Autodesk Inventor part; units mm, degrees
ref_plane "YZ Plane" through (0, 0, 0) normal (1, 0, 0) x (0, 1, 0)
ref_plane "XZ Plane" through (0, 0, 0) normal (0, 1, 0) x (-1, 0, 0)
ref_plane "XY Plane" through (0, 0, 0) normal (0, 0, 1) x (1, 0, 0)
sketch "Эскиз1" plane through (0, 0, 0) normal (0, 0, 1) x (1, 0, 0)
  line L0 (123.2502, 86.3215) -> (123.2502, 112.3215)
  circle A0 centre (130.7502, 114.3215) radius 1.5
  circle A1 centre (130.7502, 84.3215) radius 1.5
  line L1 (132.7502, 121.8215) -> (144.7502, 121.8215)
  arc A2 (132.7502, 121.8215) -> (123.2502, 112.3215) centre (132.7502, 112.3215) ccw
  arc A3 (123.2502, 86.3215) -> (132.7502, 76.8215) centre (132.7502, 86.3215) ccw
  line L2 (138.7502, 76.8215) -> (132.7502, 76.8215)
  line L3 (138.7502, 88.4715) -> (138.7502, 76.8215)
  line L4 (138.7502, 111.4715) -> (138.7502, 98.6715)
  line L5 (144.5002, -126.5097) -> (144.5002, 144.1144)
  line L6 (138.7502, 76.8215) -> (138.7502, 121.8215)
  point P0 (0, 0)
extrude "Выдавливание1" add sketch "Эскиз1" along normal blind 4
fillet "Сопряжение1" radius 2 6 edges at (123.2502, 99.3215, 4) (126.0327, 79.604, 4) (135.7502, 76.8215, 4) (135.7502, 121.8215, 4) (126.0327, 119.039, 4) (138.7502, 99.3215, 4)
fillet "Сопряжение2" radius 2 4 edges at (138.7502, 121.8215, 1) (138.1644, 121.2357, 3.4142) (138.7502, 76.8215, 1) (138.1644, 77.4073, 3.4142)
sketch "Эскиз2" plane through (0, 0, 4) normal (0, 0, 1) x (1, 0, 0)
  circle A0 centre (130.7502, 114.3215) radius 1.5
  line L0 (130.7502, 117.5547) -> (133.5502, 115.9381)
  line L1 (133.5502, 115.9381) -> (133.5502, 112.7049)
  line L2 (133.5502, 112.7049) -> (130.7502, 111.0883)
  line L3 (130.7502, 111.0883) -> (127.9502, 112.7049)
  line L4 (127.9502, 112.7049) -> (127.9502, 115.9381)
  line L5 (127.9502, 115.9381) -> (130.7502, 117.5547)
  circle A1 centre (130.7502, 84.3215) radius 1.5
  line L6 (130.7502, 87.5547) -> (133.5502, 85.9381)
  line L7 (133.5502, 85.9381) -> (133.5502, 82.7049)
  line L8 (133.5502, 82.7049) -> (130.7502, 81.0883)
  line L9 (130.7502, 81.0883) -> (127.9502, 82.7049)
  line L10 (127.9502, 82.7049) -> (127.9502, 85.9381)
  line L11 (127.9502, 85.9381) -> (130.7502, 87.5547)
  point P0 (0, 0)
  dimension "d4" = 3
  dimension "d5" = 5.6
  dimension "d6" = 5.6
extrude "Выдавливание2" cut sketch "Эскиз2" against normal blind 2.5
properties part number "накладка на петлю"
Source: CAD feature listing. Evaluate the final solid. Frame: model axes, mm. A direction names the side the tool comes from. Give positions to 0.01 mm unless a question says otherwise; leave off trailing zeros. Order: outer loops, then holes, each group sorted by start corner. A loop starts at its lowest first (then second) coordinate and runs counter-clockwise, first axis right, second up.
(1) Section query D-D (x = 131.25). State how many separate pieces and enclosed holes the cut face has, plus the area to 3 significant figures.
(2) Access query for faces 1 (the face through (132.17, 111.91, 2.77)), 2 (the face through (123.25, 99, 1)). Directions: +Z, -Z, +X, -X, +Y, -Y. A direction counts if a zero-diameter tool reaches every point of the face in a straight line with its end or side. Return the directions, or none.
(3) Pull-direction query (Y, two-part tool) for faces 3 (the face through (134.722, 77.392, 3.399)), 4 (the face through (129.37, 81.885, 2.768)), 5 (the face through (131, 100, 0)); classes: +Y half, -Y half, draft (parallel to the pull), parting line (faces both ways), or undercut.
(4) Material intervals for line 1 along Y through (x, z) = (131.75, 1.95); line 2 along Y through (x, z) = (131.25, 3.5); line 3 along X through (y, z) = (114.5, 2.2), sorted ascending.
(5) Section query B-B (y = 110). Return the cut outline in (x, z).
(6) Section query C-C (z = 3). Return the cut outline in (x, y), plus the area to 3 significant figures.
(7) Contact query for flat-ended pins moving along their axis: P1, Ø0.8, axis at y = 114, z = 3.5, coming from the +X side; P2, Ø0.8, axis at y = 84.5, z = 2, coming from the -X side; P3, Ø1.7, axis at x = 129.5, y = 85.5, coming from the +Z side. Output: stop coordinate, or through.
(8) Section query A-A (z = 0.5). Return the cut outline in (x, y).
Outcome:
1. separate pieces: 3
1. enclosed holes: 0
1. area: 139 mm2
2. face 1: +Z
2. face 2: +Z, -Z, -X, +Y, -Y
3. face 3: -Y half
3. face 4: undercut
3. face 5: draft
4. line 1: y = 76.87 to 81.67, 86.98 to 111.67, 116.98 to 121.77
4. line 2: y = 77.63 to 81.38, 87.27 to 111.38, 117.27 to 121.02
4. line 3: x = 123.51 to 127.95, 133.55 to 138.74
5. outline: (123.25, 0) - (138.75, 0) - (138.75, 2) arc R2 ccw to (136.75, 4) - (125.25, 4) arc R2 ccw to (123.25, 2) - close
6. outline: (123.52, 86.32) arc R9.23 ccw to (132.75, 77.09) - (136.75, 77.09) arc R1.73 ccw to (138.48, 78.82) - (138.48, 119.82) arc R1.73 ccw to (136.75, 121.55) - (132.75, 121.55) arc R9.23 ccw to (123.52, 112.32) - close; hole (127.95, 82.7) - (130.75, 81.09) - (133.55, 82.7) - (133.55, 85.94) - (130.75, 87.55) - (127.95, 85.94) - close; hole (127.95, 112.7) - (130.75, 111.09) - (133.55, 112.7) - (133.55, 115.94) - (130.75, 117.55) - (127.95, 115.94) - close
6. area: 573 mm2
7. P1: stops at x = 138.42
7. P2: stops at x = 123.36
7. P3: stops at z = 1.5
8. outline: (123.25, 86.32) arc R9.5 ccw to (132.75, 76.82) - (136.75, 76.82) arc R2 ccw to (138.75, 78.82) - (138.75, 119.82) arc R2 ccw to (136.75, 121.82) - (132.75, 121.82) arc R9.5 ccw to (123.25, 112.32) - close; hole circle Ø3 at (130.75, 84.32); hole circle Ø3 at (130.75, 114.32)
